```python
from build123d import *

# Parameters (mm, degrees)
ESQUISSE1_R        = 17.7
ESQUISSE1_R_2      = 12.7
BOSS_EXTRU_1_DEPTH = 8.3
ESQUISSE2_R        = 38
ESQUISSE2_R_2      = 11.2
BOSS_EXTRU_2_DEPTH = 47.8
CHANFREIN3_SIZE    = 11.200084029
CHANFREIN3_SIZE_2  = 49.8
SKETCH7_R          = 38
SKETCH7_R_2        = 26
CUT_EXTRUDE2_DEPTH = 3
CIRPATTERN1_COUNT  = 4
CIRPATTERN2_COUNT  = 3
LPATTERN1_COUNT    = 8
LPATTERN1_PITCH    = 5


with BuildPart() as part:
    # Esquisse1 → Boss.-Extru.1 (new body)
    with BuildSketch(Plane.XY):
        with Locations(Location((0, 0, 0), (0, 0, 180))):
            Circle(ESQUISSE1_R)
        with Locations(Location((0, 0, 0), (0, 0, 180))):
            Circle(ESQUISSE1_R_2, mode=Mode.SUBTRACT)
    extrude(amount=BOSS_EXTRU_1_DEPTH)

    # Esquisse2 → Boss.-Extru.2 (add)
    with BuildSketch(Plane(origin=(0, 0, 0), x_dir=(-1, 0, 0), z_dir=(0, 0, -1))):
        with Locations(Location((0, 0, 0), (0, 0, 180))):
            Circle(ESQUISSE2_R)
        with Locations(Location((0, 0, 0), (0, 0, 180))):
            Circle(ESQUISSE2_R_2, mode=Mode.SUBTRACT)
    extrude(amount=BOSS_EXTRU_2_DEPTH)

    # Chanfrein3
    # the kernel refuses this chamfer: 49.8, 11.200084029 mm, written as the material it takes off along each edge
    with BuildSketch(Plane(origin=(0, 0, -47.8), x_dir=(1, 0, 0), z_dir=(0, 1, 0))) as chanfrein3_piece_1:
        Polygon((11.2 + CHANFREIN3_SIZE, 0), (11.2, -CHANFREIN3_SIZE_2), (11.2, 0), align=None)
    revolve(axis=Axis((0, 0, -47.8), (0, 0, -1)), mode=Mode.SUBTRACT)

    # Sketch7 → Cut-Extrude2 (cut)
    with BuildSketch(Plane.XY):
        Circle(SKETCH7_R)
        Circle(SKETCH7_R_2, mode=Mode.SUBTRACT)
    cut_extrude2 = extrude(amount=-CUT_EXTRUDE2_DEPTH, mode=Mode.SUBTRACT)

    # Sketch19 → #4-40 Tapped Hole1 (revolve, cut)
    with BuildSketch(Plane(origin=(0, -30, -47.8), x_dir=(0, 1, 0), z_dir=(1, 0, 0))):
        Polygon((0, 0), (0, 5.679152758), (1.1303, 5), (1.1303, 0), align=None)
    f_4_40_tapped_hole1 = revolve(axis=Axis((0, -30, -54.15), (0, 0, 1)), mode=Mode.SUBTRACT)

    # CirPattern1: #4-40 Tapped Hole1 ×4 about axis
    cirpattern1_axis = Axis((0, 0, 0), (0, 0, 1))
    for i in range(1, CIRPATTERN1_COUNT):
        add(f_4_40_tapped_hole1.rotate(cirpattern1_axis, i * 360 / CIRPATTERN1_COUNT), mode=Mode.SUBTRACT)

    # Sketch22 → #4-40 Tapped Hole2 (revolve, cut)
    with BuildSketch(Plane(origin=(0, -15.35, 8.3), x_dir=(0, -1, 0), z_dir=(1, 0, 0))):
        Polygon((0, 0), (0, 5.679152758), (1.1303, 5), (1.1303, 0), align=None)
    f_4_40_tapped_hole2 = revolve(axis=Axis((0, -15.35, 14.65), (0, 0, -1)), mode=Mode.SUBTRACT)

    # CirPattern2: #4-40 Tapped Hole2 ×3 about axis
    cirpattern2_axis = Axis((0, 0, 0), (0, 0, 1))
    for i in range(1, CIRPATTERN2_COUNT):
        add(f_4_40_tapped_hole2.rotate(cirpattern2_axis, i * 360 / CIRPATTERN2_COUNT), mode=Mode.SUBTRACT)

    # LPattern1: Cut-Extrude2 ×8
    with Locations(*[(0, 0, -i * LPATTERN1_PITCH) for i in range(1, LPATTERN1_COUNT)]):
        add(cut_extrude2, mode=Mode.SUBTRACT)


solid = part.part
```
Could you check a few things on this model? Use its own coordinates, in mm. A direction names the side the tool comes from. Coordinates: 2 decimals unless noted, no trailing zeros. Loops run counter-clockwise (first coordinate to the right, second up) from the corner with the lowest first, then second, coordinate; pieces in that order, holes last.
1) Will these pins go through, and if not, where does the flat tip stop? pin 1 Ø3 at (x, z) = (-30.5, -2.5) entering from +Y; pin 2 Ø6 at (y, z) = (8, -23) entering from +X; pin 3 Ø8 at (x, z) = (-14, -6) entering from -Y.
Reported:
pin 1: stops at y = 24.45
pin 2: stops at x = 37.67
pin 3: stops at y = -36.63
2) Which directions (+Z, -Z, +X, -X, +Y, -Y) give clear straight access to the entire face, cutting with the end or side of a thin tool? Please do faces 1 (the face through (-0.05, -31.13, -45.33)), 2 (the face through (-8.238, 37.096, -3.986)), 3 (the face through (-20.633, -15.821, -36.479)), 4 (the face through (-5.86, 11.267, 4.092)).
Reported:
face 1: -Z
face 2: +Z, -Z
face 3: none
face 4: +Z
3) Please list where these lines run through material, in increasing order: line 1 along Z through (x, y) = (5, 22); line 2 along X through (y, z) = (4, -6); line 3 along X through (y, z) = (9, -17.5).
Reported:
line 1: z = -47.8 to 0
line 2: x = -25.69 to -12.37, 12.37 to 25.69
line 3: x = -24.39 to -12.72, 12.72 to 24.39
4) Imagine slicing it at A-A (z = -2). List the corners of the cut face in (x, y) for me.
Reported:
outline: circle Ø52 at (0, 0); hole circle Ø24.2 at (0, 0)
5) Thinking about a two-plate mould opening in X: for faces 5 (the face through (-0.01, -15.15, 2.74)), 6 (the face through (-8.238, 37.096, -23.986)), 7 (the face through (25, -8, -30)), which applies, released by +X, released by -X, zero draft, split by the parting line, or undercut?
Reported:
face 5: undercut
face 6: split by the parting line
face 7: zero draft
